```python
from build123d import *

# Parameters (mm, degrees)
CUT_EXTRUDE1_DEPTH      = 63.353829072
CIRPATTERN1_COUNT       = 4
CUT_EXTRUDE2_DEPTH      = 61.728905976
CUT_EXTRUDE2_DEPTH_BACK = 61.728905976
SKETCH4_R               = 12


with BuildPart() as part:
    # Sketch1 → Revolve1 (revolve)
    with BuildSketch(Plane.XY, mode=Mode.PRIVATE) as revolve1_sk:
        Polygon((0, 9), (0, 0), (26, 0), (36, 36), (26.659229154, 36), (19.159229154, 9), align=None)
    revolve(revolve1_sk.sketch.rotate(Axis((0, 0, 0), (0, 1, 0)), 90), axis=Axis((0, 0, 0), (0, 1, 0)))

    # Sketch2 → Cut-Extrude1 (cut, symmetric)
    with BuildSketch(Plane(origin=(0, 0, 0), x_dir=(0, 0, -1), z_dir=(1, 0, 0))):
        with BuildLine():
            Line((-10, 36), (10, 36))
            ThreePointArc((10, 36), (0, 26), (-10, 36))
        make_face()
    cut_extrude1 = extrude(amount=CUT_EXTRUDE1_DEPTH, both=True, mode=Mode.SUBTRACT)

    # CirPattern1: Cut-Extrude1 ×4 about axis
    cirpattern1_axis = Axis((0, 0, 0), (0, -1, 0))
    for i in range(1, CIRPATTERN1_COUNT):
        add(cut_extrude1.rotate(cirpattern1_axis, i * 360 / CIRPATTERN1_COUNT), mode=Mode.SUBTRACT)

    # Sketch4 → Cut-Extrude2 (cut, two sides: drawn at the far end of the back side and taken through both)
    with BuildSketch(Plane.XZ.offset(-CUT_EXTRUDE2_DEPTH_BACK)):
        with Locations(Location((0, 0, 0), (0, 0, 270))):
            Circle(SKETCH4_R)
    extrude(amount=CUT_EXTRUDE2_DEPTH + CUT_EXTRUDE2_DEPTH_BACK, mode=Mode.SUBTRACT)


solid = part.part
```
Source: CAD feature listing. Evaluate the final solid. Frame: model axes, mm. A direction names the side the tool comes from. Coordinates: 2 decimals unless noted, no trailing zeros. Write each loop counter-clockwise with the first axis right and the second up, starting at its lowest first coordinate (ties: lowest second). Pieces come first, ordered by that corner, then holes. Notation, with made-up numbers: (-17.75, 15.5) -> (26.25, 15.5) arc R13 ccw to (26.25, 24.5) -> close; hole circle Ø11 at (21, 26.25). An arc over 180 degrees is marked (long way). Return JSON: item names as keys, results as strings. Group by question number.
1) Section query C-C, the plane y = 15.5. Return loops of the section in (x, z).
2) Ray query, line 1 along X through (y, z) = (19, -9); line 2 along Z through (x, y) = (15.5, 16.5); line 3 along Y through (x, z) = (0.5, 13). Return the intervals inside material, ascending.
3) Set-up query: faces 4 (the face through (13, 9, 0)), 5 (the face through (5.4, 0, 11.2)). Return all of +Z, -Z, +X, -X, +Y, -Y with unobstructed straight access to the full face (end or side cutting, diameter ignored); none if empty.
4) Section query A-A, the plane x = 0. Return loops of the section in (y, z).
5) Contact query for flat-ended pins moving along their axis: P1, Ø10, axis at y = 8, z = 14.5, coming from the -X side; P2, Ø5, axis at y = 26.5, z = -25.5, coming from the +X side; P3, Ø6, axis at y = 28.5, z = 13, coming from the +X side; P4, Ø19, axis at x = 0, z = 0, coming from the -Y side. Output: stop coordinate, or through.
6) Section query B-B, the plane z = 0. Return loops of the section in (x, y).
7) Mould query, pull axis X, two halves, no side actions, for faces 1 (the face through (0, 26, 29)), 2 (the face through (-22, 36, -22)), 3 (the face through (-8.665, 10.252, -27.516)). Classes: +X half, -X half, draft (parallel to the pull), parting line (faces both ways), or undercut.
8) Section query D-D, the plane y = 5. Return loops of the section in (x, z), plus the area to 3 significant figures.
From the geometry:
{
 "1": {"outline": "circle Ø60.61 at (0, 0); hole circle Ø41.93 at (0, 0)"},
 "2": {"line 1": "-29.95 to -20.01, 20.01 to 29.95", "line 2": "-26.36 to -14.53, 14.53 to 26.36", "line 3": "0 to 9"},
 "3": {"face 4": "+Y", "face 5": "+Z, -Z, +X, -X, -Y"},
 "4": {"outline": "(0, -26) -> (26, -33.22) -> (26, -23.88) -> (9, -19.16) -> (9, -12) -> (0, -12) -> close; (0, 12) -> (9, 12) -> (9, 19.16) -> (26, 23.88) -> (26, 33.22) -> (0, 26) -> close"},
 "5": {"P1": "x = -27.09", "P2": "x = 24.35", "P3": "x = 32.75", "P4": "through"},
 "6": {"outline": "(-33.22, 26) -> (-26, 0) -> (-12, 0) -> (-12, 9) -> (-19.16, 9) -> (-23.88, 26) -> close; (12, 0) -> (26, 0) -> (33.22, 26) -> (23.88, 26) -> (19.16, 9) -> (12, 9) -> close"},
 "7": {"face 1": "undercut", "face 2": "draft", "face 3": "parting line"},
 "8": {"outline": "circle Ø54.78 at (0, 0); hole circle Ø24 at (0, 0)", "area": "1,900 mm²"}
}
